from build123d import *

# Parameters (mm, degrees)
SKETCH_1_R          = 4
EXTRUDE_1_DEPTH     = 4
CUT_EXTRUDE_1_DEPTH = 2


with BuildPart() as part:
    # 草图1 → 凸台-拉伸1 (new body, symmetric)
    with BuildSketch(Plane(origin=(0, 0, 0), x_dir=(0, 0, -1), z_dir=(1, 0, 0))):
        with BuildLine():
            Line((-40, 8), (40, 8))
            ThreePointArc((40, 8), (48, 0), (40, -8))
            Line((40, -8), (-40, -8))
            ThreePointArc((-40, -8), (-48, 0), (-40, 8))
        make_face()
        with Locations((40, 0)):
            Circle(SKETCH_1_R, mode=Mode.SUBTRACT)
        with Locations((-40, 0)):
            Circle(SKETCH_1_R, mode=Mode.SUBTRACT)
    extrude(amount=EXTRUDE_1_DEPTH, both=True)

    # 草图7 → 切除-拉伸1 (cut)
    with BuildSketch(Plane.ZY.offset(4)):
        with BuildLine():
            Line((-27.5, 5), (27.5, 5))
            ThreePointArc((27.5, 5), (32.5, 0), (27.5, -5))
            Line((27.5, -5), (-27.5, -5))
            ThreePointArc((-27.5, -5), (-32.5, 0), (-27.5, 5))
        make_face()
    cut_extrude_1 = extrude(amount=-CUT_EXTRUDE_1_DEPTH, mode=Mode.SUBTRACT)

    # 镜向1: 切除-拉伸1 across plane
    add(cut_extrude_1.mirror(Plane(origin=(0, 0, 0), x_dir=(0, 0, 1), z_dir=(1, 0, 0))), mode=Mode.SUBTRACT)


solid = part.part
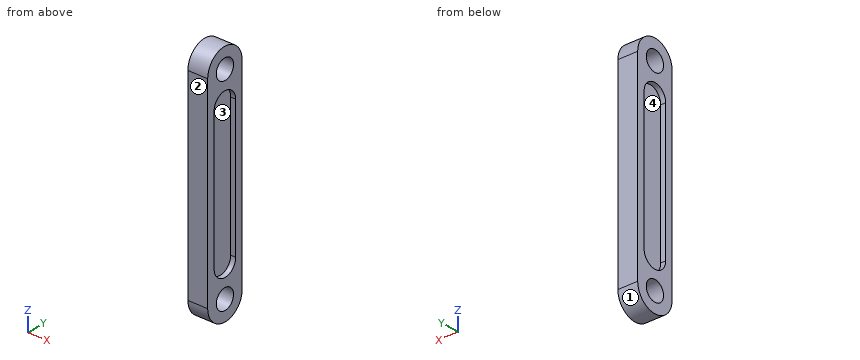
For this review, take the finished solid that the model builds, in its own axes (mm). Face numbers are marked on the shaded views. Give positions to 0.01 mm unless a question says otherwise; leave off trailing zeros. Order: outer loops, then holes, each group sorted by start corner. A loop starts at its lowest first (then second) coordinate and runs counter-clockwise, first axis right, second up. Notation, with made-up numbers: (-33, 44.25) -> (24, 44.25) arc R27 ccw to (24, 66.25) -> close; hole circle Ø9 at (-19.5, 3). An arc over 180 degrees is marked (long way). Write item = value, one per line.
1) We need section D-D, the plane x = 1. Give the boundary of the cut face in (y, z).
Findings:
outline = (-8, -40) arc R8 ccw to (8, -40) -> (8, 40) arc R8 ccw to (-8, 40) -> close; hole circle Ø8 at (0, -40); hole circle Ø8 at (0, 40)
2) To check wall thickness, follow L1, parallel to Y at x = -3.5, z = -25; L2, parallel to Y at x = -1.75, z = 40; L3, parallel to Z at x = 0.25, y = 2.5. State the ranges of each line that lie inside material, in increasing order. Write a range as from..to.
Findings:
L1 = -8..-5, 5..8
L2 = -8..-4, 4..8
L3 = -47.6..-43.12, -36.88..36.88, 43.12..47.6
3) Draft analysis for pull direction Z (two halves, no side actions). For the marked faces 1, 2, 3 and 4, state which applies: pulls with the +Z half, pulls with the -Z half, needs draft (parallel to the pull), parting line crosses it, or undercut.
Findings:
face_1 = pulls with the -Z half
face_2 = needs draft
face_3 = undercut
face_4 = undercut
4) Insertion check: pin 1 (6.5 mm diameter, centred on y = 0, z = 40, fed in from -X); pin 2 (6 mm diameter, centred on y = -1, z = 27, fed in from -X); pin 3 (1.5 mm diameter, centred on x = 0.5, y = -3.5, fed in from +Z). Each pin has a flat end and moves straight along its axis. Give the tip position at first contact, or say it passes through.
Findings:
pin_1 = through
pin_2 = -2
pin_3 = 47.51
5) We need section B-B, the plane x = -3. Give the boundary of the cut face in (y, z), and give its area (3 significant figures).
Findings:
outline = (-8, -40) arc R8 ccw to (8, -40) -> (8, 40) arc R8 ccw to (-8, 40) -> close; hole (-5, -27.5) arc R5 ccw to (5, -27.5) -> (5, 27.5) arc R5 ccw to (-5, 27.5) -> close; hole circle Ø8 at (0, -40); hole circle Ø8 at (0, 40)
area = 752 mm^2
6) We need section C-C, the plane z = 41. Give the boundary of the cut face in (x, y).
Findings:
outline = (-4, -7.94) -> (4, -7.94) -> (4, -3.87) -> (-4, -3.87) -> close; (-4, 3.87) -> (4, 3.87) -> (4, 7.94) -> (-4, 7.94) -> close
7) We need section A-A, the plane y = 0. Give the boundary of the cut face in (x, z), and give its area (3 significant figures).
Findings:
outline = (-4, -48) -> (4, -48) -> (4, -44) -> (-4, -44) -> close; (-4, -36) -> (4, -36) -> (4, -32.5) -> (2, -32.5) -> (2, 32.5) -> (4, 32.5) -> (4, 36) -> (-4, 36) -> (-4, 32.5) -> (-2, 32.5) -> (-2, -32.5) -> (-4, -32.5) -> close; (-4, 44) -> (4, 44) -> (4, 48) -> (-4, 48) -> close
area = 380 mm^2
